Here's the drawing with two shaded views (mm, measured from the low corner). I have some questions. A direction names the side the tool comes from. Give positions to 0.01 mm unless a question says otherwise; leave off trailing zeros. Order: outer loops, then holes, each group sorted by start corner. A loop starts at its lowest first (then second) coordinate and runs counter-clockwise, first axis right, second up. Notation, with made-up numbers: M 35,66.5 L 71,66.5 A17 ccw 71,72.5 Z; hole C -37.75,17 d5. An arc over 180 degrees is marked long. Use a Markdown table: item, result. Add a question column.
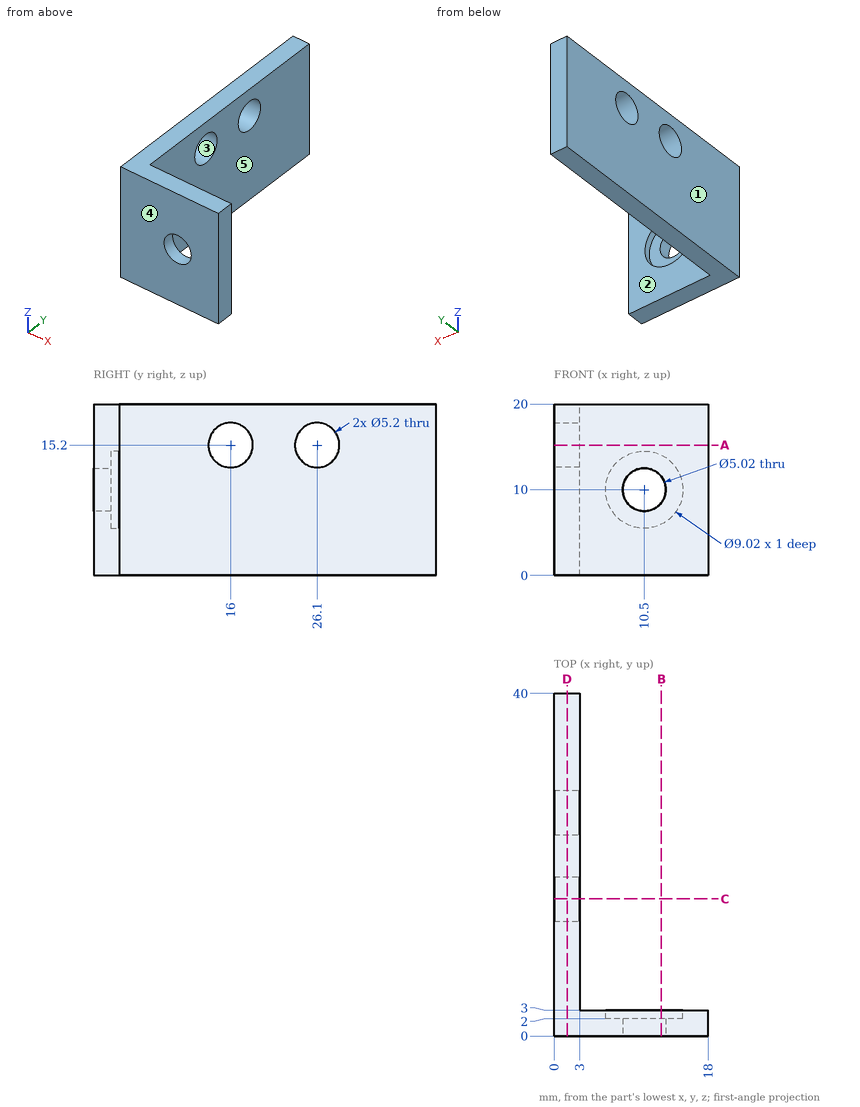
1) Suppose I cut it at B-B on x = 12.5. Please give me the cut outline in (y, z), and give its area (3 significant figures).
2) Suppose I cut it at A-A on z = 15.2. Please give me the cut outline in (x, y).
3) We'd pull the mould along Y, two halves only. Please class the marked faces 1, 2 and 3: pulls with the +Y half, pulls with the -Y half, needs draft (parallel to the pull), parting line crosses it, or undercut.
4) Suppose I cut it at C-C on y = 16. Please give me the cut outline in (x, z).
5) Suppose I cut it at D-D on x = 1.5. Please give me the cut outline in (y, z).
6) For the marked faces 4 and 5, which set-ups out of +Z, -Z, +X, -X, +Y, -Y let a thin tool reach every point of the face, with its end or its side?
7) Please list where these lines run through material, in increasing order: line 1 (Y direction, x = 1.45, z = 15.2); line 2 (Z direction, x = 10.5, y = 0.5); line 3 (X direction, y = 0.8, z = 10). Write a range as from..to.
8) For pin 1 (8 mm diameter, centred on x = 14, y = 9, fed in from -Z); pin 2 (6 mm diameter, centred on y = 26.1, z = 15.2, fed in from +X); pin 3 (5 mm diameter, centred on x = 11, z = 18, fed in from +Y); pin 4 (4 mm diameter, centred on y = 34.5, z = 2.5, fed in from -X), each with a flat end and sliding along its axis, tell me the tip position at first contact or that it passes through.
Values found:
| question | item | result |
|---|---|---|
| 1 | outline | M 0,0 L 3,0 L 3,5.96 L 2,5.96 L 2,8.48 L 0,8.48 Z; M 0,11.52 L 2,11.52 L 2,14.04 L 3,14.04 L 3,20 L 0,20 Z |
| 1 | area | 45.8 mm^2 |
| 2 | outline | M 0,0 L 18,0 L 18,3 L 3,3 L 3,13.4 L 0,13.4 Z; M 0,18.6 L 3,18.6 L 3,23.5 L 0,23.5 Z; M 0,28.7 L 3,28.7 L 3,40 L 0,40 Z |
| 3 | face 1 | needs draft |
| 3 | face 2 | pulls with the +Y half |
| 3 | face 3 | undercut |
| 4 | outline | M 0,0 L 3,0 L 3,12.6 L 0,12.6 Z; M 0,17.8 L 3,17.8 L 3,20 L 0,20 Z |
| 5 | outline | M 0,0 L 40,0 L 40,20 L 0,20 Z; hole C 16,15.2 d5.2; hole C 26.1,15.2 d5.2 |
| 6 | face 4 | +Z, -Z, +X, -X, -Y |
| 6 | face 5 | +Z, -Z, +X, +Y |
| 7 | line 1 | y = 0..13.4, 18.6..23.5, 28.7..40 |
| 7 | line 2 | z = 0..7.49, 12.51..20 |
| 7 | line 3 | x = 0..7.99, 13.01..18 |
| 8 | pin 1 | passes through |
| 8 | pin 2 | stops at x = 3 |
| 8 | pin 3 | stops at y = 3 |
| 8 | pin 4 | stops at x = 0 |
